Verification items for the finished model (mm, model axes). Face numbers are marked on the shaded views. A direction names the side the tool comes from. Round coordinates to 2 decimals unless told otherwise and drop trailing zeros. Order: outer loops, then holes, each group sorted by start corner. A loop starts at its lowest first (then second) coordinate and runs counter-clockwise, first axis right, second up. Notation, with made-up numbers: M 88.25,-14 L 99.25,-14 A17 cw 99.25,13 Z; hole C 76,42 d10. An arc over 180 degrees is marked long. One line per item, written item: value. Start each with the question number.
from build123d import *

# Parameters (mm, degrees)
F0_R     = 6
F1_DEPTH = 4
F2_R     = 4.5
F3_DEPTH = 4.5
F4_R     = 6
F4_R_2   = 4.5
F5_DEPTH = 4
F6_R     = 1.5
F7_DEPTH = 15
F8_SIZE  = 1.49999
F9_R     = 0.1


# Not quite as in the source:
# - a fillet or chamfer is up to 0.001 mm smaller than in the source, because OpenCascade refuses the exact size


with BuildPart() as f1:
    # F0 (on Front) → F1 (new body)
    with BuildSketch(Plane.XZ):
        Circle(F0_R)
    extrude(amount=F1_DEPTH)

    # F2 (on face) → F3 (join)
    with BuildSketch(Plane.XZ.offset(4)):
        Circle(F2_R)
    extrude(amount=F3_DEPTH)

    # F4 (on face) → F5 (join)
    with BuildSketch(Plane.XZ.offset(8.5)):
        Circle(F4_R)
        Circle(F4_R_2, mode=Mode.SUBTRACT)
        Circle(F4_R_2)
    extrude(amount=F5_DEPTH)

    # F6 (on face) → F7 (cut)
    with BuildSketch(Plane.XZ.offset(12.5)):
        Circle(F6_R)
    extrude(amount=-F7_DEPTH, mode=Mode.SUBTRACT)

    # F8 (size 1.5 in the source; OpenCascade refuses exactly that, so slightly less here)
    f8_edges = [f1.edges().sort_by_distance(p)[0] for p in [
        (-6, -8.5, 0),
        (-6, -4, 0),
    ]]
    chamfer(f8_edges, length=F8_SIZE)

    # F9
    f9_edges = [f1.edges().sort_by_distance(p)[0] for p in [
        (-6, -12.5, 0),
        (-6, 0, 0),
    ]]
    fillet(f9_edges, radius=F9_R)


solid = f1.part
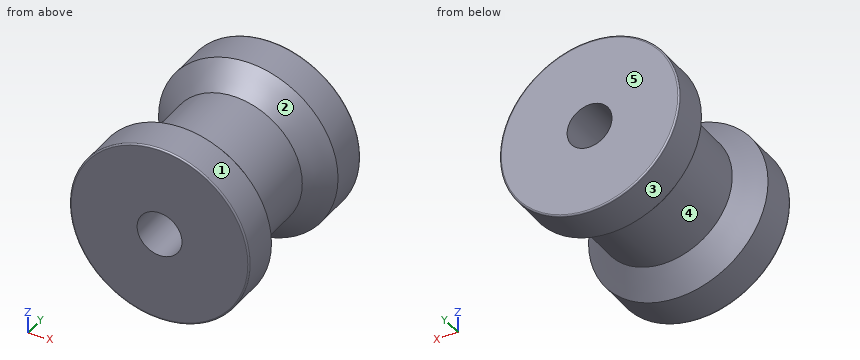
1. Section check C-C (y = -8.25). Record the cut outline in (x, z), and give its area (3 significant figures).
2. Depth check by flat-ended pin: pin 1 (6 mm diameter, centred on y = -4.5, z = 1.5, fed in from +X); pin 2 (1 mm diameter, centred on x = 2.5, y = -10.5, fed in from -Z); pin 3 (5 mm diameter, centred on y = -6, z = 2.5, fed in from +X); pin 4 (3 mm diameter, centred on y = -5, z = -4.5, fed in from -X). Enter the tip coordinate at first touch or a pass-through.
3. Scan lines: line 1 along Z through (x, y) = (0, -2.25); line 2 along Z through (x, y) = (0, -5.5); line 3 along Y through (x, z) = (5, -1.25). Record each from-to range of solid material in increasing order.
4. Tool access check on the marked faces 1 and 2. Record the directions out of +Z, -Z, +X, -X, +Y, -Y that give a thin tool (end or side, any length) a straight path to the whole face; none if there is none.
5. Draft check along Y on the marked faces 3, 4 and 5. Enter one of: released by +Y, released by -Y, zero draft, split by the parting line, or undercut.
6. Section check D-D (y = -2). Record the cut outline in (x, z).
Geometry check:
1. outline: C 0,0 d9; hole C 0,0 d3
1. area: 56.5 mm²
2. pin 1: stops at x = 6
2. pin 2: stops at z = -5.66
2. pin 3: stops at x = 4.56
2. pin 4: stops at x = -3.35
3. line 1: z = -6 to -1.5, 1.5 to 6
3. line 2: z = -4.5 to -1.5, 1.5 to 4.5
3. line 3: y = -12.5 to -9.15, -3.35 to 0
4. face 1: +Y, -Y
4. face 2: none
5. face 3: zero draft
5. face 4: undercut
5. face 5: released by +Y
6. outline: C 0,0 d12; hole C 0,0 d3
